Autodesk Inventor part; units mm, degrees
ref_plane "YZ Plane" through (0, 0, 0) normal (1, 0, 0) x (0, 1, 0)
ref_plane "XZ Plane" through (0, 0, 0) normal (0, 1, 0) x (-1, 0, 0)
ref_plane "XY Plane" through (0, 0, 0) normal (0, 0, 1) x (1, 0, 0)
sketch "Szkic1" plane through (0, 0, 0) normal (0, 0, 1) x (1, 0, 0)
  line L0 (0, 0) -> (57, 0)
  line L1 (57, 0) -> (57, 74)
  line L2 (57, 74) -> (0, 74)
  line L3 (0, 74) -> (0, 0)
  line L4 (28.5, 74) -> (28.5, 67) construction
  line L5 (0, 37) -> (4.5, 37) construction
  line L6 (28.5, 0) -> (28.5, 7) construction
  line L7 (57, 37) -> (52.5, 37) construction
  line L8 (4.5, 7) -> (52.5, 7)
  line L9 (52.5, 7) -> (52.5, 67)
  line L10 (52.5, 67) -> (4.5, 67)
  line L11 (4.5, 67) -> (4.5, 7)
  line L12 (57, 0) -> (49, 0) construction
  line L13 (0, 0) -> (8, 0) construction
  line L14 (8, 0) -> (8, 4) construction
  line L15 (49, 0) -> (49, 4) construction
  circle A0 centre (49, 4) radius 1.55
  circle A1 centre (8, 4) radius 1.55
  line L16 (57, 74) -> (49, 74) construction
  line L17 (49, 74) -> (49, 70) construction
  line L18 (0, 74) -> (8, 74) construction
  line L19 (8, 74) -> (8, 70) construction
  circle A2 centre (8, 70) radius 1.55
  circle A3 centre (49, 70) radius 1.55
  dimension "d0" = 57
  dimension "d1" = 74
  dimension "d2" = 7
  dimension "d3" = 4.5
  dimension "d4" = 7
  dimension "d5" = 4.5
  dimension "d6" = 8
  dimension "d7" = 8
  dimension "d8" = 4
  dimension "d9" = 3.1
  dimension "d10" = 3.1
  dimension "d11" = 4
  dimension "d12" = 3.1
  dimension "d13" = 3.1
extrude "Wyciągnięcie proste1" add sketch "Szkic1" along normal blind 4
properties part number "Uzupelnienie_podwozia"
CAD build for the part. Positions are in the model's coordinates, mm. A direction names the side the tool comes from. Round coordinates to 2 decimals unless told otherwise and drop trailing zeros. Order: outer loops, then holes, each group sorted by start corner. A loop starts at its lowest first (then second) coordinate and runs counter-clockwise, first axis right, second up. Notation, with made-up numbers: (41.25, -26) - (70.25, -26) arc R19 ccw to (70.25, -1) - close; hole circle Ø3 at (9.25, -10). An arc over 180 degrees is marked (long way). Answer in a Markdown table with one row per item. Add a question column.
(1) Mould opens along X. For faces 1 (the face through (4.5, 37, 2)), 2 (the face through (28, 0, 2)), 3 (the face through (52.5, 37, 2)), 4 (the face through (0, 38, 2)) say: +X half, -X half, draft (parallel to the pull), parting line (faces both ways), or undercut.
(2) Drop a flat-ended pin along its axis: pin 1 Ø3 at (x, y) = (8, 70) entering from +Z. Give the stop position or say it passes through.
(3) 3-axis set-ups, long thin cutter, end or side, ignore diameter. For faces 5 (the face through (28, 7, 2)), 6 (the face through (53, 38, 4)): which of +Z, -Z, +X, -X, +Y, -Y reach the whole face in a straight line?
(4) Band-saw the part on C-C on y = 4. List the corners of the cut face in (x, z), and give its area (3 significant figures).
(5) Band-saw the part on B-B on x = 25. List the corners of the cut face in (y, z), and give its area (3 significant figures).
(6) Band-saw the part on A-A on y = 48. List the corners of the cut face in (x, z).
(7) Band-saw the part on D-D on z = 3.4. List the corners of the cut face in (x, y), and give its area (3 significant figures).
(8) Probe L1, parallel to X at y = 70, z = 1.6; L2, parallel to Y at x = 8, z = 1.5; L3, parallel to X at y = 14, z = 0.8. List the from-to ranges inside material, lowest first. Write a range as [from, to].
Data:
| question | item | result |
|---|---|---|
| 1 | face 1 | undercut |
| 1 | face 2 | draft |
| 1 | face 3 | undercut |
| 1 | face 4 | -X half |
| 2 | pin 1 | passes through |
| 3 | face 5 | +Z, -Z |
| 3 | face 6 | +Z, +X, -X, +Y, -Y |
| 4 | outline | (0, 0) - (6.45, 0) - (6.45, 4) - (0, 4) - close; (9.55, 0) - (47.45, 0) - (47.45, 4) - (9.55, 4) - close; (50.55, 0) - (57, 0) - (57, 4) - (50.55, 4) - close |
| 4 | area | 203 mm^2 |
| 5 | outline | (0, 0) - (7, 0) - (7, 4) - (0, 4) - close; (67, 0) - (74, 0) - (74, 4) - (67, 4) - close |
| 5 | area | 56.0 mm^2 |
| 6 | outline | (0, 0) - (4.5, 0) - (4.5, 4) - (0, 4) - close; (52.5, 0) - (57, 0) - (57, 4) - (52.5, 4) - close |
| 7 | outline | (0, 0) - (57, 0) - (57, 74) - (0, 74) - close; hole (4.5, 7) - (52.5, 7) - (52.5, 67) - (4.5, 67) - close; hole circle Ø3.1 at (8, 4); hole circle Ø3.1 at (8, 70); hole circle Ø3.1 at (49, 4); hole circle Ø3.1 at (49, 70) |
| 7 | area | 1,310 mm^2 |
| 8 | L1 | x = [0, 6.45], [9.55, 47.45], [50.55, 57] |
| 8 | L2 | y = [0, 2.45], [5.55, 7], [67, 68.45], [71.55, 74] |
| 8 | L3 | x = [0, 4.5], [52.5, 57] |
